```python
from build123d import *

# Parameters (mm, degrees)
SKETCH1_W           = 52.6
SKETCH1_H           = 11
SKETCH2_R           = 5
BOSS_EXTRUDE1_DEPTH = 1.35
SKETCH3_R           = 3.5
BOSS_EXTRUDE2_DEPTH = 1.8
SKETCH4_R           = 2
BOSS_EXTRUDE3_DEPTH = 11.7
CUT_EXTRUDE1_REACH  = 71.221
HOLE1_D             = 1.95
HOLE1_DEPTH         = 6.5
HOLE2_D             = 1.95
HOLE2_DEPTH         = 6.5
HOLE3_D             = 1.95
HOLE3_DEPTH         = 6.5
HOLE4_D             = 7
HOLE4_DEPTH         = 6.4
HOLE5_D             = 2.1
HOLE5_DEPTH         = 3
HOLE6_D             = 2.1
HOLE6_DEPTH         = 3
HOLE7_D             = 2.1
HOLE7_DEPTH         = 3
SKETCH25_R          = 11
BOSS_EXTRUDE4_DEPTH = 36.83


with BuildPart() as part:
    # Sketch1 → Revolve1 (revolve)
    with BuildSketch(Plane.XY, mode=Mode.PRIVATE) as revolve1_sk:
        with Locations((26.3, 5.5)):
            Rectangle(SKETCH1_W, SKETCH1_H)
    revolve(revolve1_sk.sketch.rotate(Axis((0, 0, 0), (1, 0, 0)), 270), axis=Axis((0, 0, 0), (1, 0, 0)))

    # Sketch2 → Boss-Extrude1 (add)
    with BuildSketch(Plane.ZY):
        with Locations(Location((0, 0, 0), (0, 0, 180))):
            Circle(SKETCH2_R)
    extrude(amount=BOSS_EXTRUDE1_DEPTH)

    # Sketch3 → Boss-Extrude2 (add)
    with BuildSketch(Plane.ZY.offset(1.35)):
        Circle(SKETCH3_R)
    extrude(amount=BOSS_EXTRUDE2_DEPTH)

    # Sketch4 → Boss-Extrude3 (add)
    with BuildSketch(Plane.ZY.offset(3.15)):
        Circle(SKETCH4_R)
    extrude(amount=BOSS_EXTRUDE3_DEPTH)

    # Cut-Extrude1: up to this plane
    cut_extrude1_end = Plane(origin=(-3.675, 0, 3.675), z_dir=(0.707106781186547, 0, -0.707106781186548))
    # Sketch6 → Cut-Extrude1 (cut, up to the surface)
    with BuildSketch(Plane.ZY.offset(14.85), mode=Mode.PRIVATE) as cut_extrude1_sk1:
        with BuildLine():
            Line((1.5, 1.322875656), (1.5, -1.322875656))
            ThreePointArc((1.5, -1.322875656), (2, 0), (1.5, 1.322875656))
        make_face()
    cut_extrude1_tool1 = split(extrude(cut_extrude1_sk1.sketch, amount=-CUT_EXTRUDE1_REACH, mode=Mode.PRIVATE), bisect_by=cut_extrude1_end, keep=Keep.BOTH, mode=Mode.PRIVATE)
    add(cut_extrude1_tool1.solids().sort_by_distance((-14.85, 0, 1.702311))[0], mode=Mode.SUBTRACT)

    # Hole1
    with Locations(Plane.ZY):
        with Locations((7, 0)):
            Hole(HOLE1_D / 2, depth=HOLE1_DEPTH)

    # Hole2
    with Locations(Plane.ZY):
        with Locations((-3.5, -6.062177826)):
            Hole(HOLE2_D / 2, depth=HOLE2_DEPTH)

    # Hole3
    with Locations(Plane.ZY):
        with Locations((-3.5, 6.062177826)):
            Hole(HOLE3_D / 2, depth=HOLE3_DEPTH)

    # Hole4
    with Locations(Plane(origin=(52.6, 0, 0), x_dir=(0, 0, -1), z_dir=(1, 0, 0))):
        with Locations((0, 0)):
            Hole(HOLE4_D / 2, depth=HOLE4_DEPTH)

    # Hole5
    with Locations(Plane(origin=(52.6, 0, 0), x_dir=(0, 0, -1), z_dir=(1, 0, 0))):
        with Locations((-8.5, 0)):
            Hole(HOLE5_D / 2, depth=HOLE5_DEPTH)

    # Hole6
    with Locations(Plane(origin=(52.6, 0, 0), x_dir=(0, 0, -1), z_dir=(1, 0, 0))):
        with Locations((4.25, -7.361215932)):
            Hole(HOLE6_D / 2, depth=HOLE6_DEPTH)

    # Hole7
    with Locations(Plane(origin=(52.6, 0, 0), x_dir=(0, 0, -1), z_dir=(1, 0, 0))):
        with Locations((4.25, 7.361215932)):
            Hole(HOLE7_D / 2, depth=HOLE7_DEPTH)

    # Sketch25 → Boss-Extrude4 (add)
    with BuildSketch(Plane(origin=(52.6, 0, 0), x_dir=(0, 0, -1), z_dir=(1, 0, 0))):
        Circle(SKETCH25_R)
    extrude(amount=BOSS_EXTRUDE4_DEPTH)


solid = part.part
```
The listing builds one solid part. Answer for the finished solid, in the listing's coordinates (mm). A direction names the side the tool comes from. Coordinates: 2 decimals unless noted, no trailing zeros. Loops run counter-clockwise (first coordinate to the right, second up) from the corner with the lowest first, then second, coordinate; pieces in that order, holes last. Notation, with made-up numbers: (41.5, 76) -> (48.5, 76) arc R4 cw to (48.5, 83) -> close; hole circle Ø3 at (23, 18.5). An arc over 180 degrees is marked (long way). Return JSON: item names as keys, results as strings. Group by question number.
(1) Determine the mould class of faces 1 (the cylindrical face through (49.355, -1.341, 3.233)), 2 (the flat face through (-14.85, 0, 0)), 3 (the cylindrical face through (-1, 0, 5)) for opening direction Y: released by +Y, released by -Y, zero draft, split by the parting line, or undercut.
(2) A cutting plane is placed at A-A on y = 0. Count the separate pieces of the cut face and the enclosed holes in it, and give its area (3 significant figures).
(3) A cutting plane is placed at C-C on x = 14.5. Write down the section's boundary in (y, z).
(4) A cutting plane is placed at B-B on z = 0. Write down the section's boundary in (x, y).
(5) Find the intervals of material crossed by probe 1 along Y at (x, z) = (2.75, -3.5); probe 2 along X at (y, z) = (-0.25, 6.75); probe 3 along X at (y, z) = (-2.5, 3.25), in increasing order. Write a range as from..to.
(6) Given pin 1 Ø5 at (x, z) = (29, -7) entering from -Y; pin 2 Ø0.6 at (y, z) = (0.5, 7) entering from -X; pin 3 Ø1 at (x, z) = (57, -1) entering from -Y, each flat-ended and moving along its own axis, determine where each tip first touches the part or whether it passes through.
(7) Which of the six approach directions +Z, -Z, +X, -X, +Y, -Y give full straight-line access (tool end or side, diameter ignored) to faces 4 (the flat face through (-1.35, 2.2, -3.3)), 5 (the flat face through (-10, 0, 1.5)), 6 (the flat face through (49.6, 0, 8)), 7 (the flat face through (89.43, 0, 0))?
The answers:
{
 "1": {"face 1": "undercut", "face 2": "zero draft", "face 3": "split by the parting line"},
 "2": {"separate pieces": "1", "enclosed holes": "2", "area": "1,970 mm^2"},
 "3": {"outline": "circle Ø22 at (0, 0)"},
 "4": {"outline": "(-14.85, -2) -> (-3.15, -2) -> (-3.15, -3.5) -> (-1.35, -3.5) -> (-1.35, -5) -> (0, -5) -> (0, -11) -> (89.43, -11) -> (89.43, 11) -> (0, 11) -> (0, 5) -> (-1.35, 5) -> (-1.35, 3.5) -> (-3.15, 3.5) -> (-3.15, 2) -> (-14.85, 2) -> close; hole (46.2, -3.5) -> (52.6, -3.5) -> (52.6, 3.5) -> (46.2, 3.5) -> close"},
 "5": {"probe 1": "y = -10.43..-7.04, -5.09..5.09, 7.04..10.43", "probe 2": "x = 6.5..89.43", "probe 3": "x = -1.35..89.43"},
 "6": {"pin 1": "stops at y = -10.04", "pin 2": "stops at x = 6.5", "pin 3": "stops at y = -10.99"},
 "7": {"face 4": "-X", "face 5": "+Z, -X, +Y, -Y", "face 6": "none", "face 7": "+Z, -Z, +X, +Y, -Y"}
}
